from build123d import *

# Parameters (mm, degrees)
SKETCH1_R           = 11.925
SKETCH1_R_2         = 1
BOSS_EXTRUDE1_DEPTH = 2


with BuildPart() as part:
    # Sketch1 → Boss-Extrude1 (new body)
    with BuildSketch(Plane(origin=(0, 0, 0), x_dir=(1, 0, 0), z_dir=(0, 1, 0))):
        with Locations(Location((0, 0, 0), (0, 0, 270))):
            Circle(SKETCH1_R)
        with Locations(Location((9.925, 0, 0), (0, 0, 270))):
            Circle(SKETCH1_R_2, mode=Mode.SUBTRACT)
        with BuildLine():
            ThreePointArc((-1.9898224, -9.723488665), (-7.018034803, -7.018034803), (-9.723488665, -1.9898224))
            ThreePointArc((-9.723488665, -1.9898224), (-7.925, 0), (-9.723488665, 1.9898224))
            ThreePointArc((-9.723488665, 1.9898224), (-7.018034803, 7.018034803), (-1.9898224, 9.723488665))
            ThreePointArc((-1.9898224, 9.723488665), (0, 7.925), (1.9898224, 9.723488665))
            ThreePointArc((1.9898224, 9.723488665), (7.018034803, 7.018034803), (9.723488665, 1.9898224))
            ThreePointArc((9.723488665, 1.9898224), (7.925, 0), (9.723488665, -1.9898224))
            ThreePointArc((9.723488665, -1.9898224), (7.018034803, -7.018034803), (1.9898224, -9.723488665))
            ThreePointArc((1.9898224, -9.723488665), (0, -7.925), (-1.9898224, -9.723488665))
        make_face(mode=Mode.SUBTRACT)
        with Locations(Location((-9.925, 0, 0), (0, 0, 270))):
            Circle(SKETCH1_R_2, mode=Mode.SUBTRACT)
        with Locations(Location((0, -9.925, 0), (0, 0, 270))):
            Circle(SKETCH1_R_2, mode=Mode.SUBTRACT)
        with Locations(Location((0, 9.925, 0), (0, 0, 270))):
            Circle(SKETCH1_R_2, mode=Mode.SUBTRACT)
    extrude(amount=BOSS_EXTRUDE1_DEPTH)


solid = part.part
Input: part model. Units: mm. Frame: model coordinates. A direction names the side the tool comes from. Coordinates: 2 decimals unless noted, no trailing zeros. Order: outer loops, then holes, each group sorted by start corner. A loop starts at its lowest first (then second) coordinate and runs counter-clockwise, first axis right, second up. Notation, with made-up numbers: M 11.5,-22 L 30.5,-22 A18 cw 30.5,-10 Z; hole C -16.5,69 d9. An arc over 180 degrees is marked long. Write item = value, one per line. Start each with the question number.
(1) Section B-B on x = 0. Output: boundary loops of the cut face in (y, z) (3 decimals), and give its area (3 significant figures).
(2) Section C-C on x = 2.5. Output: boundary loops of the cut face in (y, z).
(3) Line query: line 1 along X through (y, z) = (0.9, 0.25); line 2 along X through (y, z) = (0.2, -8.5); line 3 along X through (y, z) = (0.4, -3). Output: solid intervals per line, ascending. Write a range as [from, to].
(4) Reachability of faces 4 (the flat face through (-9, 0, -1)), 5 (the cylindrical face through (-7.075, 0.986, -6.96)) from +Z, -Z, +X, -X, +Y, -Y: full face, straight path, thin tool, end or side. Return the list, or none.
(5) Section D-D on z = 7. Output: boundary loops of the cut face in (x, y).
(6) First-contact query: P1, Ø2.5, axis at x = 0, z = -9.925, coming from the -Y side; P2, Ø1, axis at y = 1.5, z = -9, coming from the -X side. Flat tips, straight axial feed; report the tip coordinate or a pass-through.
(7) Section A-A on z = 0. Output: boundary loops of the cut face in (x, y) (3 decimals).
(8) Pull-direction query (X, two-part tool) for faces 1 (the cylindrical face through (3.582, 0.986, 11.374)), 2 (the cylindrical face through (8.95, 0.99, -0.22)), 3 (the flat face through (-9, 2, -1)); classes: released by +X, released by -X, zero draft, split by the parting line, or undercut.
Result set:
q1.outline = M 0,-11.925 L 2,-11.925 L 2,-10.925 L 0,-10.925 Z; M 0,-8.925 L 2,-8.925 L 2,-7.925 L 0,-7.925 Z; M 0,7.925 L 2,7.925 L 2,8.925 L 0,8.925 Z; M 0,10.925 L 2,10.925 L 2,11.925 L 0,11.925 Z
q1.area = 8.00 mm²
q2.outline = M 0,-11.66 L 2,-11.66 L 2,-9.6 L 0,-9.6 Z; M 0,9.6 L 2,9.6 L 2,11.66 L 0,11.66 Z
q3.line_1 = [-11.92, -10.89], [-8.96, -7.94], [7.94, 8.96], [10.89, 11.92]
q3.line_2 = [-8.36, -5.12], [-1.4, 1.4], [5.12, 8.36]
q3.line_3 = [-11.54, -9.46], [9.46, 11.54]
q4.face_4 = +Z, -Z, +X, -X, -Y
q4.face_5 = +Y, -Y
q5.outline = M -9.65,0 L -7.04,0 L -7.04,2 L -9.65,2 Z; M 7.04,0 L 9.65,0 L 9.65,2 L 7.04,2 Z
q6.P1 = 0
q6.P2 = -8.36
q7.outline = M -11.925,0 L -10.925,0 L -10.925,2 L -11.925,2 Z; M -8.925,0 L -7.925,0 L -7.925,2 L -8.925,2 Z; M 7.925,0 L 8.925,0 L 8.925,2 L 7.925,2 Z; M 10.925,0 L 11.925,0 L 11.925,2 L 10.925,2 Z
q8.face_1 = split by the parting line
q8.face_2 = undercut
q8.face_3 = zero draft
